Can you work these out from the drawing? Everything is in mm from the part's minimum corner. Round coordinates to 2 decimals unless told otherwise and drop trailing zeros. Order: outer loops, then holes, each group sorted by start corner. A loop starts at its lowest first (then second) coordinate and runs counter-clockwise, first axis right, second up. Notation, with made-up numbers: (74.5, 21) -> (97.5, 21) arc R15 cw to (97.5, 39) -> close; hole circle Ø9 at (-38, 86.5). An arc over 180 degrees is marked (long way). One line per item, written item: value.
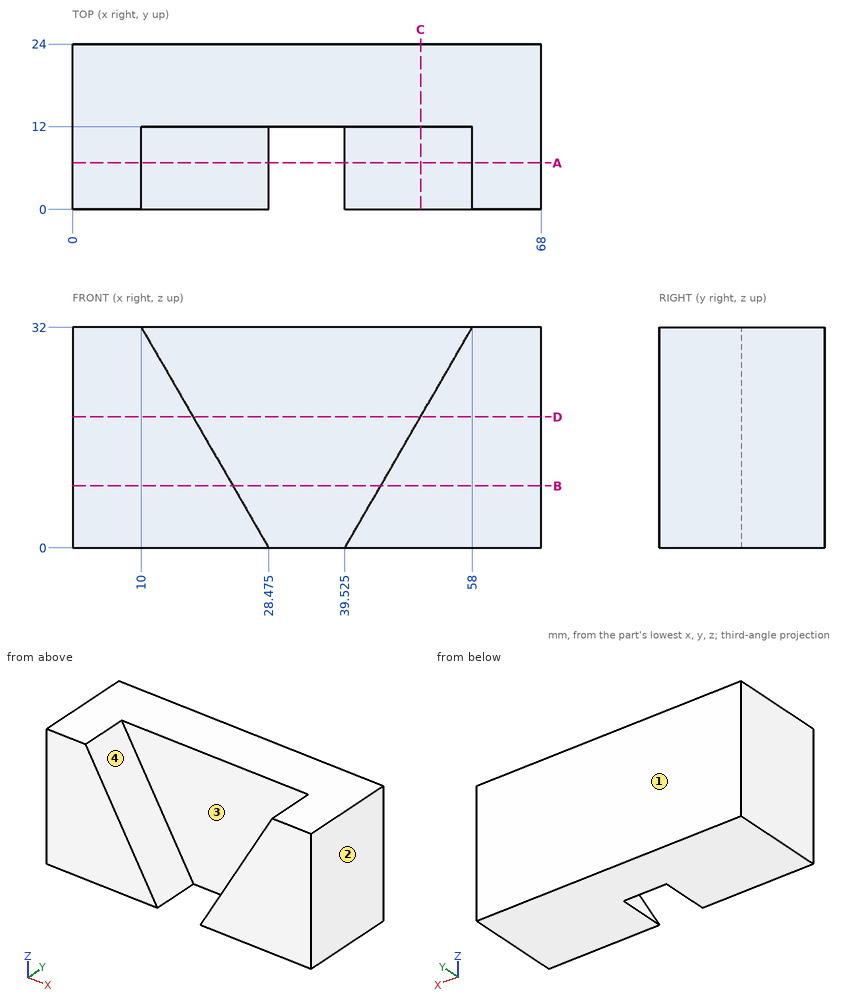
Q1. Will this pin go through, and if not, where does the flat tip stop? pin 1 Ø12 at (x, z) = (26, 18) entering from -Y.
Answers below:
pin 1: y = 12
Q2. Please list where these lines run through material, in increasing order: line 1 along Y through (x, z) = (30, 30.5); line 2 along X through (y, z) = (2.75, 3.5) (1 decimal); line 3 along X through (y, z) = (3.5, 23).
Answers below:
line 1: 12 to 24
line 2: 0 to 26.5, 41.5 to 68
line 3: 0 to 15.2, 52.8 to 68
Q3. I want a section at C-C on x = 50.5. List the corners of the cut face in (y, z) for me.
Answers below:
outline: (0, 0) -> (24, 0) -> (24, 32) -> (12, 32) -> (12, 19.01) -> (0, 19.01) -> close
Q4. I want a section at D-D on z = 19. List the corners of the cut face in (x, y) for me, plus the area to 3 significant figures.
Answers below:
outline: (0, 0) -> (17.51, 0) -> (17.51, 12) -> (50.49, 12) -> (50.49, 0) -> (68, 0) -> (68, 24) -> (0, 24) -> close
area: 1,240 mm^2
Q5. I want a section at A-A on y = 6.75. List the corners of the cut face in (x, z) for me (1 decimal).
Answers below:
outline: (0, 0) -> (28.5, 0) -> (10, 32) -> (0, 32) -> close; (39.5, 0) -> (68, 0) -> (68, 32) -> (58, 32) -> close
Q6. We'd pull the mould along X, two halves only. Please class the marked faces 1, 2, 3 and 4: released by +X, released by -X, zero draft, split by the parting line, or undercut.
Answers below:
face 1: zero draft
face 2: released by +X
face 3: undercut
face 4: undercut
Q7. I want a section at B-B on z = 9. List the corners of the cut face in (x, y) for me, plus the area to 3 significant figures.
Answers below:
outline: (0, 0) -> (23.28, 0) -> (23.28, 12) -> (44.72, 12) -> (44.72, 0) -> (68, 0) -> (68, 24) -> (0, 24) -> close
area: 1,370 mm^2
